```python
from build123d import *

# Parameters (mm, degrees)
SKETCH1_W                = 15.88
SKETCH1_H                = 12.7
BOSS_EXTRUDE1_DEPTH      = 8.255
BOSS_EXTRUDE2_DEPTH      = 14.2
BOSS_EXTRUDE2_DEPTH_BACK = 11
SKETCH2_R                = 4
CHAMFER1_SIZE            = 3
CHAMFER1_SIZE2           = 1.595128295
SKETCH4_R                = 1
BOSS_EXTRUDE3_DEPTH      = 0.5
SKETCH5_R                = 2.153363707
CUT_EXTRUDE1_DEPTH       = 27.9918622


with BuildPart() as part:
    # Sketch1 → Boss-Extrude1 (new body)
    with BuildSketch(Plane(origin=(0, 0, 0), x_dir=(1, 0, 0), z_dir=(0, 1, 0))):
        Rectangle(SKETCH1_W, SKETCH1_H)
    extrude(amount=BOSS_EXTRUDE1_DEPTH)

    # Sketch2 → Boss-Extrude2 (add, two sides: drawn at the far end of the back side and taken through both)
    with BuildSketch(Plane(origin=(0, 8.255, 0), x_dir=(1, 0, 0), z_dir=(0, 1, 0)).offset(-BOSS_EXTRUDE2_DEPTH_BACK)):
        with Locations(Location((2.917, 0, 0), (0, 0, 270))):
            Circle(SKETCH2_R)
    extrude(amount=BOSS_EXTRUDE2_DEPTH + BOSS_EXTRUDE2_DEPTH_BACK)

    # Chamfer1
    chamfer1_edges = [part.edges().sort_by_distance(p)[0] for p in [
        (2.917, -2.745, -4),
    ]]
    chamfer1_side = [part.faces().sort_by_distance(p)[0] for p in [
        (2.917, -2.745, 0),
    ]]
    chamfer(chamfer1_edges, length=CHAMFER1_SIZE, length2=CHAMFER1_SIZE2, reference=chamfer1_side[0])

    # Sketch4 → Boss-Extrude3 (add)
    with BuildSketch(Plane.XZ.offset(2.745)):
        with Locations(Location((2.917, 0, 0), (0, 0, 90))):
            Circle(SKETCH4_R)
    extrude(amount=BOSS_EXTRUDE3_DEPTH)

    # Sketch5 → Cut-Extrude1 (cut, through all)
    with BuildSketch(Plane(origin=(0, 0, -6.35), x_dir=(-1, 0, 0), z_dir=(0, 0, -1))):
        with Locations((4.13, 4.1275)):
            Circle(SKETCH5_R)
    extrude(amount=-CUT_EXTRUDE1_DEPTH, mode=Mode.SUBTRACT)


solid = part.part
```
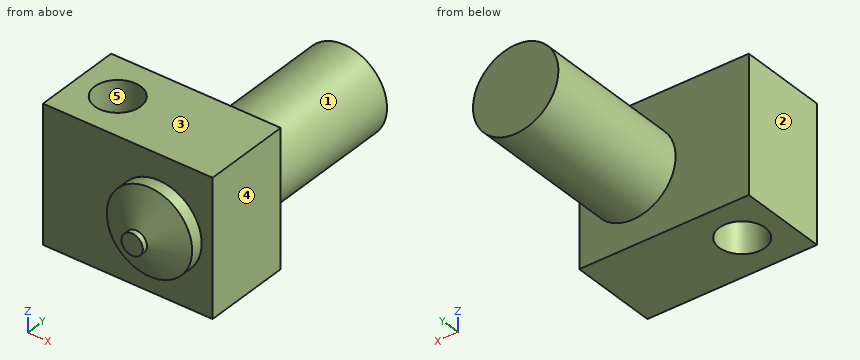
The listing builds one solid part. Answer for the finished solid, in the listing's coordinates (mm). Face numbers are marked on the shaded views. A direction names the side the tool comes from. Coordinates: 2 decimals unless noted, no trailing zeros. Loops run counter-clockwise (first coordinate to the right, second up) from the corner with the lowest first, then second, coordinate; pieces in that order, holes last. Notation, with made-up numbers: M -37,57.5 L 19,57.5 A24 ccw 19,83.5 Z; hole C 12.5,43 d2. An arc over 180 degrees is marked long. Answer as a JSON object with one key per item and string values. Group by question number.
Item 1: Section B-B (y = 6) is taken. Write down the section's boundary in (x, z).
Item 2: Which of the six approach directions +Z, -Z, +X, -X, +Y, -Y give full straight-line access (tool end or side, diameter ignored) to the marked faces 1 and 2?
Item 3: Consider L1, parallel to Y at x = -4.13, z = 3 (3 decimals); L2, parallel to X at y = 5.5, z = -2; L3, parallel to Y at x = 5.5, z = 4.75 (3 decimals). Determine where each line is inside the solid, lowest interval first.
Item 4: Section C-C (z = 0) is taken. Write down the section's boundary in (x, y) (1 decimal), and give its area (3 significant figures).
Item 5: Determine the mould class of the marked faces 3, 4 and 5 for opening direction X: +X half, -X half, draft (parallel to the pull), parting line (faces both ways), or undercut.
Item 6: Section A-A (x = -4.13) is taken. Write down the section's boundary in (y, z) (3 decimals), and give its area (3 significant figures).
Item 7: Section D-D (z = -5) is taken. Write down the section's boundary in (x, y) (1 decimal).
Item 8: Each of these flat-tipped pins is pushed along its axis until it touches: P1, Ø5, axis at y = 14, z = -3, coming from the +X side; P2, Ø1.5, axis at x = 0, z = 2, coming from the -Y side; P3, Ø5, axis at x = -5.5, z = -3, coming from the +Y side (3 decimals). Where does it stop, or does it pass through?
Solved:
{
 "1": {"outline": "M -7.94,-6.35 L -5.19,-6.35 L -5.19,6.35 L -7.94,6.35 Z; M -3.07,-6.35 L 7.94,-6.35 L 7.94,6.35 L -3.07,6.35 Z"},
 "2": {"face 1": "+Y", "face 2": "+Z, -Z, -X, +Y, -Y"},
 "3": {"L1": "y = 0 to 1.974, 6.281 to 8.255", "L2": "x = -7.94 to -5.79, -2.47 to 7.94", "L3": "y = 0 to 8.255"},
 "4": {"outline": "M -7.9,0 L -1.1,0 L -1.1,-1.1 L 1.9,-2.7 L 1.9,-3.2 L 3.9,-3.2 L 3.9,-2.7 L 6.9,-1.1 L 6.9,0 L 7.9,0 L 7.9,8.3 L 6.9,8.3 L 6.9,22.5 L -1.1,22.5 L -1.1,8.3 L -7.9,8.3 Z; hole C -4.1,4.1 d4.3", "area": "248 mm2"},
 "5": {"face 3": "draft", "face 4": "+X half", "face 5": "undercut"},
 "6": {"outline": "M 0,-6.35 L 1.974,-6.35 L 1.974,6.35 L 0,6.35 Z; M 6.281,-6.35 L 8.255,-6.35 L 8.255,6.35 L 6.281,6.35 Z", "area": "50.1 mm2"},
 "7": {"outline": "M -7.9,0 L 7.9,0 L 7.9,8.3 L -7.9,8.3 Z; hole C -4.1,4.1 d4.3"},
 "8": {"P1": "stops at x = 6.89", "P2": "stops at y = -1.79", "P3": "stops at y = 8.255"}
}
